from build123d import *

# Parameters (mm, degrees)
EXTRUDE_1_DEPTH = 30
SKETCH_4_R      = 2
EXTRUDE_2_DEPTH = 10
M4X0_7_1_D      = 3.3
M4X0_7_1_DEPTH  = 10.1
M4X0_7_1_TIP    = 0.991420021


with BuildPart() as part:
    # 草圖1 → 填料-伸長1 (new body)
    with BuildSketch(Plane.XY):
        Polygon((-2.020725942, 3.5), (-4.041451884, 0), (-2.020725942, -3.5), (2.020725942, -3.5), (4.041451884, 0), (2.020725942, 3.5), align=None)
    extrude(amount=EXTRUDE_1_DEPTH)

    # 草圖4 → 填料-伸長2 (add)
    with BuildSketch(Plane(origin=(0, 0, 0), x_dir=(-1, 0, 0), z_dir=(0, 0, -1))):
        Circle(SKETCH_4_R)
    extrude(amount=EXTRUDE_2_DEPTH)

    # M4x0.7 螺紋孔1
    with Locations(Plane.XY.offset(30)):
        with Locations((0, 0)):
            Hole(M4X0_7_1_D / 2, depth=M4X0_7_1_DEPTH)
            with Locations((0, 0, -(M4X0_7_1_DEPTH + M4X0_7_1_TIP / 2))):  # 118° drill point
                Cone(0, M4X0_7_1_D / 2, M4X0_7_1_TIP, mode=Mode.SUBTRACT)


solid = part.part
Could you check a few things on this model? Use its own coordinates, in mm. A direction names the side the tool comes from. Give positions to 0.01 mm unless a question says otherwise; leave off trailing zeros. Order: outer loops, then holes, each group sorted by start corner. A loop starts at its lowest first (then second) coordinate and runs counter-clockwise, first axis right, second up.
1. Suppose I cut it at D-D (z = -5). List the corners of the cut face in (x, y) for me.
2. Will these pins go through, and if not, where does the flat tip stop? P1, Ø1, axis at x = 3, z = 4, coming from the -Y side; P2, Ø4, axis at y = 0.5, z = 13.5, coming from the -X side.
3. For faces 5 (the flat face through (3.045, 1.726, 14.79)), 6 (the cylindrical face through (0, -2, -5)), which set-ups out of +Z, -Z, +X, -X, +Y, -Y let a thin tool reach every point of the face, with its end or its side?
4. We'd pull the mould along Y, two halves only. Please class faces 1 (the flat face through (2, 0, 30)), 2 (the flat face through (-3, 1.8, 14.8)), 3 (the cylindrical face through (1.216, 1.115, 24.879)), 4 (the flat face through (0, -3.5, 15)): pulls with the +Y half, pulls with the -Y half, needs draft (parallel to the pull), parting line crosses it, or undercut.
5. Suppose I cut it at C-C (y = -2.5). List the corners of the cut face in (x, z) for me, plus the area to 3 significant figures.
6. Suppose I cut it at B-B (z = 5). List the corners of the cut face in (x, y) for me.
7. Suppose I cut it at A-A (z = 27.5). List the corners of the cut face in (x, y) for me.
8. I need wall thicknesses on L1, parallel to Y at x = 0, z = 24.75; L2, parallel to Z at x = -2.25, y = 1; L3, parallel to X at y = -0.25, z = 23.5. Which ranges of each line are inside material? Lowest first, please.
Solved:
1. outline: circle Ø4 at (0, 0)
2. P1: stops at y = -2.67
2. P2: stops at x = -4.04
3. face 5: +Z, -Z, +X, +Y
3. face 6: -Z
4. face 1: needs draft
4. face 2: pulls with the +Y half
4. face 3: undercut
4. face 4: pulls with the -Y half
5. outline: (-2.6, 0) - (2.6, 0) - (2.6, 30) - (-2.6, 30) - close
5. area: 156 mm2
6. outline: (-4.04, 0) - (-2.02, -3.5) - (2.02, -3.5) - (4.04, 0) - (2.02, 3.5) - (-2.02, 3.5) - close
7. outline: (-4.04, 0) - (-2.02, -3.5) - (2.02, -3.5) - (4.04, 0) - (2.02, 3.5) - (-2.02, 3.5) - close; hole circle Ø3.3 at (0, 0)
8. L1: y = -3.5 to -1.65, 1.65 to 3.5
8. L2: z = 0 to 30
8. L3: x = -3.9 to -1.63, 1.63 to 3.9
